Source: CAD feature listing. Evaluate the final solid. Frame: model axes, mm. A direction names the side the tool comes from. Give positions to 0.01 mm unless a question says otherwise; leave off trailing zeros. Order: outer loops, then holes, each group sorted by start corner. A loop starts at its lowest first (then second) coordinate and runs counter-clockwise, first axis right, second up. Notation, with made-up numbers: M 52.5,82.5 L 92.5,82.5 A24 cw 92.5,121.5 Z; hole C 71.25,57 d2. An arc over 180 degrees is marked long. Use CSV: the item, a comma, the result in double quotes. Start each with the question number.
1. Section query B-B, the plane x = -4. Return the cut outline in (y, z) (3 decimals), plus the area to 3 significant figures.
2. Pin query (flat end, axial travel): P1, Ø1, axis at y = 17, z = 15, coming from the +X side; P2, Ø7.5, axis at x = 7, z = 17.5, coming from the -Y side; P3, Ø3, axis at y = 27, z = 6.5, coming from the -X side. Return the tip coordinate at first contact, or that it passes through.
3. Line query: line 1 along X through (y, z) = (8.5, 20); line 2 along Y through (x, z) = (19, 2.5) (3 decimals); line 3 along Y through (x, z) = (5.5, 13.5) (3 decimals). Output: solid intervals per line, ascending. Write a range as [from, to].
4. Section query C-C, the plane z = 12.7. Return the cut outline in (x, y) (3 decimals).
5. Section query D-D, the plane y = 22.5. Return the cut outline in (x, z).
6. Reachability of faces 5 (the flat face through (3, 15.875, 4)), 6 (the flat face through (2, 9, 13)), 7 (the flat face through (2, 10, 25.4)) from +Z, -Z, +X, -X, +Y, -Y: full face, straight path, thin tool, end or side. Return the list, or none.
7. Mould query, pull axis X, two halves, no side actions, for faces 1 (the flat face through (-10.19, 4, 13)), 2 (the flat face through (15.21, 5, 13)), 3 (the flat face through (21.21, 8, 13)), 4 (the flat face through (-16.19, 8, 13)). Classes: released by +X, released by -X, zero draft, split by the parting line, or undercut.
8. Section query A-A, the plane z = 22.25. Return the cut outline in (x, y) (3 decimals), plus the area to 3 significant figures.
from build123d import *

# Parameters (mm, degrees)
BOSS_EXTRUDE1_DEPTH = 25.4
SKETCH2_R           = 8.5
BOSS_EXTRUDE2_DEPTH = 14.5


with BuildPart() as part:
    # Sketch1 → Boss-Extrude1 (new body)
    with BuildSketch(Plane.XY):
        Polygon((-10.189534884, 0), (-10.189534884, 9), (15.210465116, 9), (15.210465116, 0), (21.210465116, 0), (21.210465116, 15.875), (-16.189534884, 15.875), (-16.189534884, 0), align=None)
    extrude(amount=BOSS_EXTRUDE1_DEPTH)

    # Sketch2 → Boss-Extrude2 (add)
    with BuildSketch(Plane(origin=(0, 15.875, 0), x_dir=(1, 0, 0), z_dir=(0, 1, 0))):
        with Locations((2.510465116, -12.7)):
            Circle(SKETCH2_R)
    extrude(amount=BOSS_EXTRUDE2_DEPTH)


solid = part.part
Result set:
1,outline,"M 9,0 L 15.875,0 L 15.875,7.235 L 30.375,7.235 L 30.375,18.165 L 15.875,18.165 L 15.875,25.4 L 9,25.4 Z"
1,area,"333 mm2"
2,P1,"x = 10.82"
2,P2,"y = 9"
2,P3,"x = -4.57"
3,line 1,"[-16.19, -10.19], [15.21, 21.21]"
3,line 2,"[0, 15.875]"
3,line 3,"[9, 30.375]"
4,outline,"M -16.19,0 L -10.19,0 L -10.19,9 L 15.21,9 L 15.21,0 L 21.21,0 L 21.21,15.875 L 11.01,15.875 L 11.01,30.375 L -5.99,30.375 L -5.99,15.875 L -16.19,15.875 Z"
5,outline,"C 2.51,12.7 d17"
6,face 5,"+Y"
6,face 6,"+Z, -Z, -Y"
6,face 7,"+Z, +X, -X, +Y, -Y"
7,face 1,"undercut"
7,face 2,"undercut"
7,face 3,"released by +X"
7,face 4,"released by -X"
8,outline,"M -16.19,0 L -10.19,0 L -10.19,9 L 15.21,9 L 15.21,0 L 21.21,0 L 21.21,15.875 L -16.19,15.875 Z"
8,area,"365 mm2"
